from build123d import *

# Parameters (mm, degrees)
SKETCH1_R           = 37.5
SKETCH1_R_2         = 35
BOSS_EXTRUDE1_DEPTH = 40
SKETCH2_R           = 35
BOSS_EXTRUDE2_DEPTH = 5
SKETCH3_R           = 0.75
CUT_EXTRUDE1_DEPTH  = 5


with BuildPart() as part:
    # Sketch1 → Boss-Extrude1 (new body)
    with BuildSketch(Plane.XY):
        Circle(SKETCH1_R)
        Circle(SKETCH1_R_2, mode=Mode.SUBTRACT)
    extrude(amount=BOSS_EXTRUDE1_DEPTH)

    # Sketch2 → Boss-Extrude2 (add)
    with BuildSketch(Plane(origin=(0, 0, 0), x_dir=(-1, 0, 0), z_dir=(0, 0, -1))):
        Circle(SKETCH2_R)
    extrude(amount=-BOSS_EXTRUDE2_DEPTH)

    # Sketch3 → Cut-Extrude1 (cut)
    with BuildSketch(Plane.XY.offset(40)):
        with Locations((0, 36.25)):
            Circle(SKETCH3_R)
        with Locations((36.25, 0)):
            Circle(SKETCH3_R)
        with Locations((0, -36.25)):
            Circle(SKETCH3_R)
        with Locations((-36.25, 0)):
            Circle(SKETCH3_R)
    extrude(amount=-CUT_EXTRUDE1_DEPTH, mode=Mode.SUBTRACT)


solid = part.part
Design review of the part built by this model. Coordinates are the model's own, in mm. A direction names the side the tool comes from. Give positions to 0.01 mm unless a question says otherwise; leave off trailing zeros. Write each loop counter-clockwise with the first axis right and the second up, starting at its lowest first coordinate (ties: lowest second). Pieces come first, ordered by that corner, then holes. Notation, with made-up numbers: M -34.5,4.5 L 21.5,4.5 A21 cw 21.5,33.5 Z; hole C -28,-17.5 d3. An arc over 180 degrees is marked long. Answer as a JSON object with one key per item and string values. Group by question number.
1) Clearance check with flat-ended pins moving along their axes: pin 1 Ø1.5 at (x, z) = (-13.5, 35.5) entering from -Y; pin 2 Ø4 at (x, y) = (-22.5, -17.5) entering from +Z; pin 3 Ø6 at (x, z) = (-10.5, 18.5) entering from +Y. State where each tip first meets the part, or that it passes through.
2) We need section D-D (z = 33). Give the boundary of the cut face in (x, y), and give its area (3 significant figures).
3) For line 1 along Y through (x, z) = (0, 36); line 2 along Y through (x, z) = (0, 28); line 3 along Z through (x, y) = (23.5, -3.5), list the stretches that pass through material, from the lowest coordinate up.
4) Tool access review of faces 1 (the face through (0, 0, 5)), 2 (the face through (-31, 17, 40)): name each direction out of +Z, -Z, +X, -X, +Y, -Y from which nothing blocks a thin tool from reaching the whole face with its end or side.
5) We need section B-B (x = 2). Give the boundary of the cut face in (y, z).
6) Mouldability with a two-part tool opening along X and no side actions: class faces 3 (the face through (1, 1, 0)), 4 (the face through (-4.88, 37.18, 19.72)), 5 (the face through (-28, -21, 22)) as released by +X, released by -X, zero draft, split by the parting line, or undercut.
7) We need section C-C (y = 4). Give the boundary of the cut face in (x, z), and give its area (3 significant figures).
8) We need section A-A (z = 37.5). Give the boundary of the cut face in (x, y), and give its area (3 significant figures).
Answer key:
{
 "1": {"pin 1": "stops at y = -35.27", "pin 2": "stops at z = 5", "pin 3": "stops at y = 36.74"},
 "2": {"outline": "C 0,0 d75; hole C 0,0 d70", "area": "569 mm²"},
 "3": {"line 1": "y = -37.5 to -37, -35.5 to -35, 35 to 35.5, 37 to 37.5", "line 2": "y = -37.5 to -35, 35 to 37.5", "line 3": "z = 0 to 5"},
 "4": {"face 1": "+Z", "face 2": "+Z, +X, -X, +Y, -Y"},
 "5": {"outline": "M -37.45,0 L 37.45,0 L 37.45,40 L 34.94,40 L 34.94,5 L -34.94,5 L -34.94,40 L -37.45,40 Z"},
 "6": {"face 3": "zero draft", "face 4": "split by the parting line", "face 5": "undercut"},
 "7": {"outline": "M -37.29,0 L 37.29,0 L 37.29,40 L 34.77,40 L 34.77,5 L -34.77,5 L -34.77,40 L -37.29,40 Z", "area": "549 mm²"},
 "8": {"outline": "C 0,0 d75; hole C -36.25,0 d1.5; hole C 0,0 d70; hole C 0,-36.25 d1.5; hole C 0,36.25 d1.5; hole C 36.25,0 d1.5", "area": "562 mm²"}
}
